from build123d import *

# Parameters (mm, degrees)
F1_DEPTH    = 127
F2_R        = 4.7625
F3_DEPTH    = 25.4
F4_W        = 15.875
F4_H        = 19.05
F5_DEPTH    = 25.401
F6_R        = 4.953
F7_DEPTH    = 127.001
F8_T1_DEPTH = 76.2
F8_T3_DEPTH = 88.9


# Not quite as in the source:
# - a fillet or chamfer that OpenCascade refuses, or shapes differently, is made with other operations: its cross-section is extruded or revolved along the edge and cut away or added


with BuildPart() as f1:
    # F0 (on Right) → F1 (new body)
    with BuildSketch(Plane.YZ):
        with BuildLine():
            Line((0, 28.575), (0, 0))
            Line((0, 0), (25.4, 0))
            Line((25.4, 0), (25.4, 63.5))
            Line((25.4, 63.5), (12.7, 63.5))
            Line((12.7, 63.5), (12.7, 39.0525))
            ThreePointArc((12.7, 39.0525), (9.6312112999, 31.6437887001), (2.2225, 28.575))
            Line((2.2225, 28.575), (0, 28.575))
        make_face()
    extrude(amount=F1_DEPTH)

    # F2 (on face) → F3 (cut)
    with BuildSketch(Plane.XZ.offset(-12.7)):
        with Locations((111.125, 47.625)):
            Circle(F2_R)
        with Locations((15.875, 47.625)):
            Circle(F2_R)
    extrude(amount=-F3_DEPTH, mode=Mode.SUBTRACT)

    # F4 (on face) → F5 (cut, through all)
    with BuildSketch(Plane.XZ):
        with Locations((94.9325, 9.525)):
            Rectangle(F4_W, F4_H)
        with Locations((62.5475, 9.525)):
            Rectangle(F4_W, F4_H)
        with Locations((30.1625, 9.525)):
            Rectangle(F4_W, F4_H)
    extrude(amount=-F5_DEPTH, mode=Mode.SUBTRACT)

    # F6 (on face) → F7 (cut, through all)
    with BuildSketch(Plane.YZ.offset(127)):
        with Locations((11.684, 12.7)):
            Circle(F6_R)
    extrude(amount=-F7_DEPTH, mode=Mode.SUBTRACT)

    # F8: fillet of radius 12.7 on 4 edges, made by hand

    # F8_s2 → F8_t1 (cut)
    with BuildSketch(Plane.XZ.offset(-57.15)):
        with BuildLine():
            ThreePointArc((0, 50.8), (3.7197438789, 59.7802561211), (12.7, 63.5))
            Line((12.7, 63.5), (0, 63.5))
            Line((0, 63.5), (0, 50.8))
        make_face()
        with BuildLine():
            ThreePointArc((127, 50.8), (123.2802561211, 59.7802561211), (114.3, 63.5))
            Line((114.3, 63.5), (127, 63.5))
            Line((127, 63.5), (127, 50.8))
        make_face()
    extrude(amount=F8_T1_DEPTH, mode=Mode.SUBTRACT)

    # F8_s4 → F8_t3 (cut)
    with BuildSketch(Plane.XZ.offset(-57.15)):
        with BuildLine():
            ThreePointArc((0, 12.7), (3.7197438789, 3.7197438789), (12.7, 0))
            Line((12.7, 0), (0, 0))
            Line((0, 0), (0, 12.7))
        make_face()
        with BuildLine():
            ThreePointArc((127, 12.7), (123.2802561211, 3.7197438789), (114.3, 0))
            Line((114.3, 0), (127, 0))
            Line((127, 0), (127, 12.7))
        make_face()
    extrude(amount=F8_T3_DEPTH, mode=Mode.SUBTRACT)


solid = f1.part
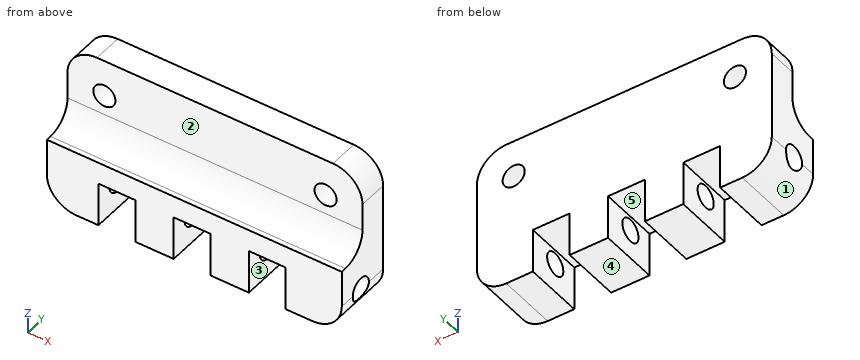
Source: CAD feature listing. Evaluate the final solid. Frame: model axes, mm. Face numbers are marked on the shaded views. A direction names the side the tool comes from. Coordinates: 2 decimals unless noted, no trailing zeros. Order: outer loops, then holes, each group sorted by start corner. A loop starts at its lowest first (then second) coordinate and runs counter-clockwise, first axis right, second up. Notation, with made-up numbers: M -29.5,30.5 L -14.5,30.5 A28 ccw -14.5,50.5 Z; hole C 37.25,-26 d6. An arc over 180 degrees is marked long. Write each question's results on one line, items separated by ' | '. Start each with the question number.
1. Material intervals for L1, parallel to X at y = 6, z = 13 (3 decimals); L2, parallel to Z at x = 32.5, y = 14.25; L3, parallel to Y at x = 102, z = 47, sorted ascending.
2. Pin query (flat end, axial travel): pin 1 (11.5 mm diameter, centred on y = 11.684, z = 12.7, fed in from +X); pin 2 (5.5 mm diameter, centred on y = 11.5, z = 12, fed in from +X); pin 3 (2.5 mm diameter, centred on x = 57, y = 1, fed in from +Z); pin 4 (8 mm diameter, centred on x = 66, y = 18, fed in from -Z). Return the tip coordinate at first contact, or that it passes through.
3. Draft query along X for the marked faces 1, 2 and 3. Return one class per face: +X half, -X half, draft (parallel to the pull), parting line (faces both ways), or undercut.
4. Section A-A, the plane x = 108.5. Return the cut outline in (y, z) (1 decimal), then the cut area to 3 significant figures.
5. Section C-C, the plane z = 10. State how many separate pieces and enclosed holes the cut face has, then the cut area to 3 significant figures.
6. Reachability of the marked faces 4 and 5 from +Z, -Z, +X, -X, +Y, -Y: full face, straight path, thin tool, end or side. Return the list, or none.
7. Section B-B, the plane x = 49.5. Return the cut outline in (y, z) (1 decimal), then the cut area to 3 significant figures.
Solution:
1) L1: 0 to 22.225, 38.1 to 54.61, 70.485 to 86.995, 102.87 to 127 | L2: 19.05 to 63.5 | L3: 12.7 to 25.4
2) pin 1: x = 127 | pin 2: through | pin 3: z = 28.58 | pin 4: z = 19.05
3) face 1: -X half | face 2: draft | face 3: undercut
4) outline: M 0,0 L 25.4,0 L 25.4,43.7 L 12.7,43.7 L 12.7,39.1 A10.5 cw 2.2,28.6 L 0,28.6 Z; M 12.7,51.6 L 25.4,51.6 L 25.4,63.5 L 12.7,63.5 Z; hole C 11.7,12.7 d9.9 | area: 1,010 mm²
5) separate pieces: 8 | enclosed holes: 0 | area: 1,350 mm²
6) face 4: -Z, +X, -X, +Y, -Y | face 5: -Z, +Y, -Y
7) outline: M 0,0 L 25.4,0 L 25.4,63.5 L 12.7,63.5 L 12.7,39.1 A10.5 cw 2.2,28.6 L 0,28.6 Z; hole C 11.7,12.7 d9.9 | area: 1,120 mm²
